```python
from build123d import *

# Parameters (mm, degrees)
SKETCH_W                 = 70.5
SKETCH_H                 = 44.45
PAD_DEPTH                = 12.7
SKETCH001_R              = 1.6
POCKET_DEPTH             = 181.311112
SKETCH001_MIRRORED_2_R   = 1.6
POCKET_MIRRORED_2_DEPTH  = 181.311112
POCKET001_DEPTH          = 11.2
CLONE001_PLACEMENT_ANGLE = 180


with BuildPart() as part:
    # Sketch → Pad (new body)
    with BuildSketch(Plane.XY):
        with Locations((-3.8, 0)):
            Rectangle(SKETCH_W, SKETCH_H)
    extrude(amount=PAD_DEPTH)

    # Sketch001 (on Face6 of Pad) → Pocket (cut, through all)
    with BuildSketch(Plane.XY.offset(12.7)):
        with Locations((-12.95, 18.55)):
            Circle(SKETCH001_R)
    pocket = extrude(amount=-POCKET_DEPTH, mode=Mode.SUBTRACT)

    # Sketch001 Mirrored 2 → Pocket Mirrored 2 (cut, through all)
    with BuildSketch(Plane(origin=(0, 0, 12.7), x_dir=(-1, 0, 0), z_dir=(0, 0, -1))):
        with Locations((-12.95, 18.55)):
            Circle(SKETCH001_MIRRORED_2_R)
    pocket_mirrored_2 = extrude(amount=POCKET_MIRRORED_2_DEPTH, mode=Mode.SUBTRACT)

    # Mirrored001: Pocket, Pocket Mirrored 2 across XZ
    add(pocket.mirror(Plane.XZ), mode=Mode.SUBTRACT)
    add(pocket_mirrored_2.mirror(Plane.XZ), mode=Mode.SUBTRACT)

    # Sketch002 (on Face4 of MultiTransform) → Pocket001 (cut)
    with BuildSketch(Plane(origin=(0, 0, 0), x_dir=(1, 0, 0), z_dir=(0, 0, -1))):
        with BuildLine():
            Line((-36.55, -19.725), (-36.55, 19.725))
            Line((-36.55, 19.725), (-17.05, 19.725))
            Line((-17.05, 19.725), (-17.05, 18.55))
            ThreePointArc((-17.05, 18.55), (-12.95, 14.45), (-8.85, 18.55))
            Line((-8.85, 19.725), (-8.85, 18.55))
            Line((-8.85, 19.725), (8.85, 19.725))
            Line((8.85, 19.725), (8.85, 18.55))
            ThreePointArc((8.85, 18.55), (12.95, 14.45), (17.05, 18.55))
            Line((17.05, 19.725), (17.05, 18.55))
            Line((31.45, 19.725), (17.05, 19.725))
            Line((31.45, 19.725), (31.45, -19.725))
            Line((31.45, -19.725), (17.05, -19.725))
            Line((17.05, -19.725), (17.05, -18.549981))
            ThreePointArc((17.05, -18.549981), (12.949999, -14.45), (8.85, -18.549983))
            Line((8.85, -19.725), (8.85, -18.549983))
            Line((-8.85, -19.725), (8.85, -19.725))
            Line((-8.85, -19.725), (-8.85, -18.55))
            ThreePointArc((-8.85, -18.55), (-12.95, -14.45), (-17.05, -18.55))
            Line((-17.05, -19.725), (-17.05, -18.55))
            Line((-36.55, -19.725), (-17.05, -19.725))
        make_face()
    extrude(amount=-POCKET001_DEPTH, mode=Mode.SUBTRACT)


with BuildPart() as part_1:
    # Clone001 placement: moved
    add(part.part.moved(Location((0, 0, 12.7))).rotate(Axis((0, 0, 12.7), (1, 0, 0)), CLONE001_PLACEMENT_ANGLE))


solid = part_1.part
```
Input: part model. Units: mm. Frame: model coordinates. A direction names the side the tool comes from. Give positions to 0.01 mm unless a question says otherwise; leave off trailing zeros. Order: outer loops, then holes, each group sorted by start corner. A loop starts at its lowest first (then second) coordinate and runs counter-clockwise, first axis right, second up. Notation, with made-up numbers: (-28.75, 71) - (12.25, 71) arc R30 cw to (12.25, 105) - close; hole circle Ø1 at (15, -30). An arc over 180 degrees is marked (long way). Put each result on its own line as item: value.
Item 1: Section query A-A, the plane x = -12.95. Return loops of the section in (y, z) (3 decimals).
Found:
outline: (-22.225, 0) - (-20.15, 0) - (-20.15, 12.7) - (-22.225, 12.7) - close; (-16.95, 0) - (16.95, 0) - (16.95, 12.7) - (14.45, 12.7) - (14.45, 1.5) - (-14.45, 1.5) - (-14.45, 12.7) - (-16.95, 12.7) - close; (20.15, 0) - (22.225, 0) - (22.225, 12.7) - (20.15, 12.7) - close
Item 2: Contact query for flat-ended pins moving along their axis: pin 1 (1.5 mm diameter, centred on x = 0, y = -7, fed in from +Z); pin 2 (2.5 mm diameter, centred on x = 12.95, y = 18.55, fed in from +Z); pin 3 (0.9 mm diameter, centred on y = 19, z = 6, fed in from +X). Output: stop coordinate, or through.
Found:
pin 1: stops at z = 1.5
pin 2: passes through
pin 3: stops at x = 17.05
Item 3: Access query for faces 1 (the flat face through (-4, -22.225, 6)), 2 (the cylindrical face through (13.04, -14.45, 7.18)), 3 (the flat face through (24, -19.725, 7)). Directions: +Z, -Z, +X, -X, +Y, -Y. A direction counts if a zero-diameter tool reaches every point of the face in a straight line with its end or side. Return the directions, or none.
Found:
face 1: +Z, -Z, +X, -X, -Y
face 2: +Z
face 3: +Z, +X
Item 4: Section query C-C, the plane y = 3.5. Return loops of the section in (x, z), then the cut area to 3 significant figures.
Found:
outline: (-39.05, 0) - (31.45, 0) - (31.45, 1.5) - (-36.55, 1.5) - (-36.55, 12.7) - (-39.05, 12.7) - close
area: 134 mm^2
Item 5: Section query D-D, the plane x = 0.5. Return loops of the section in (y, z) (3 decimals), then the cut area to 3 significant figures.
Found:
outline: (-22.225, 0) - (22.225, 0) - (22.225, 12.7) - (19.725, 12.7) - (19.725, 1.5) - (-19.725, 1.5) - (-19.725, 12.7) - (-22.225, 12.7) - close
area: 123 mm^2
Item 6: Section query B-B, the plane z = 10.75. Return loops of the section in (x, y) (3 decimals), then the cut area to 3 significant figures.
Found:
outline: (-39.05, -22.225) - (31.45, -22.225) - (31.45, -19.725) - (17.05, -19.725) - (17.05, -18.55) arc R4.1 ccw to (8.85, -18.55) - (8.85, -19.725) - (-8.85, -19.725) - (-8.85, -18.55) arc R4.1 ccw to (-17.05, -18.55) - (-17.05, -19.725) - (-36.55, -19.725) - (-36.55, 19.725) - (-17.05, 19.725) - (-17.05, 18.55) arc R4.1 ccw to (-8.85, 18.55) - (-8.85, 19.725) - (8.85, 19.725) - (8.85, 18.55) arc R4.1 ccw to (17.05, 18.55) - (17.05, 19.725) - (31.45, 19.725) - (31.45, 22.225) - (-39.05, 22.225) - close; hole circle Ø3.2 at (-12.95, -18.55); hole circle Ø3.2 at (-12.95, 18.55); hole circle Ø3.2 at (12.95, -18.55); hole circle Ø3.2 at (12.95, 18.55)
area: 563 mm^2
Item 7: Ray query, L1, parallel to X at y = -18.55, z = 6; L2, parallel to Y at x = 12.95, z = 5.5 (3 decimals); L3, parallel to Y at x = 6.5, z = 11.25 (3 decimals). Return the intervals inside material, ascending. Write a range as from..to.
Found:
L1: x = -39.05..-36.55, -17.05..-14.55, -11.35..-8.85, 8.85..11.35, 14.55..17.05
L2: y = -22.225..-20.15, -16.95..-14.45, 14.45..16.95, 20.15..22.225
L3: y = -22.225..-19.725, 19.725..22.225
Item 8: Draft query along X for faces 4 (the flat face through (-2, 0, 1.5)), 5 (the flat face through (-39.05, 0, 6)), 6 (the flat face through (-14, -15, 12.7)). Return one class per face: +X half, -X half, draft (parallel to the pull), parting line (faces both ways), or undercut.
Found:
face 4: undercut
face 5: -X half
face 6: draft
